The model under review builds one solid part; all positions refer to its coordinate system, in mm. A direction names the side the tool comes from. Round coordinates to 2 decimals unless told otherwise and drop trailing zeros. Order: outer loops, then holes, each group sorted by start corner. A loop starts at its lowest first (then second) coordinate and runs counter-clockwise, first axis right, second up. Notation, with made-up numbers: M 54.5,6.5 L 67.5,6.5 A24 cw 67.5,45.5 Z; hole C 69,24.25 d1. An arc over 180 degrees is marked long. One line per item, written item: value. Start each with the question number.
Autodesk Inventor part; units mm, degrees
ref_plane "YZ Plane" through (0, 0, 0) normal (1, 0, 0) x (0, 1, 0)
ref_plane "XZ Plane" through (0, 0, 0) normal (0, 1, 0) x (-1, 0, 0)
ref_plane "XY Plane" through (0, 0, 0) normal (0, 0, 1) x (1, 0, 0)
sketch "Sketch1" plane through (0, 0, 0) normal (0, 0, 1) x (1, 0, 0)
  line L0 (190, -75) -> (-250, -75)
  line L1 (190, 75) -> (190, -75)
  line L2 (-250, 75) -> (-235, 75)
  line L3 (-250, -75) -> (-250, 75)
  line L4 (-255, -10) -> (-255, -60)
  line L5 (-255, -60) -> (-250, -60)
  line L6 (-250, -10) -> (-250, -60)
  line L7 (-255, -10) -> (-250, -10)
  line L8 (-255, 60) -> (-255, 10)
  line L9 (-255, 10) -> (-250, 10)
  line L10 (-250, 60) -> (-250, 10)
  line L11 (-255, 60) -> (-250, 60)
  line L12 (190, 60) -> (190, 10)
  line L13 (190, 10) -> (195, 10)
  line L14 (195, 60) -> (195, 10)
  line L15 (190, 60) -> (195, 60)
  line L16 (190, -10) -> (190, -60)
  line L17 (190, -60) -> (195, -60)
  line L18 (195, -10) -> (195, -60)
  line L19 (190, -10) -> (195, -10)
  line L20 (140, 75) -> (152.5, 75)
  line L21 (20, -45) -> (55.3553, -9.6447)
  line L22 (-100, 75) -> (-78.9949, 53.9949)
  line L23 (-15.3553, -9.6447) -> (-18.8909, -13.1802)
  line L24 (-18.8909, -13.1802) -> (-40.1041, 8.033)
  line L25 (-40.1041, 8.033) -> (-36.5685, 11.5685)
  line L26 (-57.7817, 32.7817) -> (-36.5685, 11.5685)
  line L27 (-57.7817, 32.7817) -> (-61.3173, 29.2462)
  line L28 (-61.3173, 29.2462) -> (-82.5305, 50.4594)
  line L29 (-82.5305, 50.4594) -> (-78.9949, 53.9949)
  line L30 (118.9949, 53.9949) -> (140, 75)
  line L31 (118.9949, 53.9949) -> (122.5305, 50.4594)
  line L32 (122.5305, 50.4594) -> (101.3173, 29.2462)
  line L33 (101.3173, 29.2462) -> (97.7817, 32.7817)
  line L34 (76.5685, 11.5685) -> (97.7817, 32.7817)
  line L35 (76.5685, 11.5685) -> (80.1041, 8.033)
  line L36 (80.1041, 8.033) -> (58.8909, -13.1802)
  line L37 (58.8909, -13.1802) -> (55.3553, -9.6447)
  line L38 (-15.3553, -9.6447) -> (20, -45)
  line L39 (-210, 75) -> (-210, 70)
  line L40 (-210, 70) -> (-235, 70)
  line L41 (-235, 70) -> (-235, 75)
  line L42 (177.5, 75) -> (190, 75)
  line L43 (177.5, 75) -> (177.5, 70)
  line L44 (177.5, 70) -> (152.5, 70)
  line L45 (152.5, 70) -> (152.5, 75)
  line L46 (-165, 75) -> (-100, 75)
  line L47 (-165, 75) -> (-165, 70)
  line L48 (-165, 70) -> (-190, 70)
  line L49 (-190, 70) -> (-190, 75)
  line L50 (-210, 75) -> (-190, 75)
  point P0 (0, 0)
extrude "Extrusion1" add sketch "Sketch1" along normal blind 5
sketch "Sketch2" plane through (0, 0, 5) normal (0, 0, 1) x (1, 0, 0)
  point P0 (0, 0)
sketch "Sketch4" plane through (0, 0, 5) normal (0, 0, 1) x (1, 0, 0)
  line L0 (190, -60) -> (195, -60)
  line L1 (195, -60) -> (195, -10)
  line L2 (195, -10) -> (190, -10)
  line L3 (190, -10) -> (190, 10)
  line L4 (190, 10) -> (195, 10)
  line L5 (195, 10) -> (195, 60)
  line L6 (195, 60) -> (190, 60)
  line L7 (190, 60) -> (190, 75)
  line L8 (190, 75) -> (177.5, 75)
  line L9 (177.5, 75) -> (177.5, 70)
  line L10 (177.5, 70) -> (152.5, 70)
  line L11 (152.5, 70) -> (152.5, 75)
  line L12 (152.5, 75) -> (140, 75)
  line L13 (140, 75) -> (118.9949, 53.9949)
  line L14 (118.9949, 53.9949) -> (122.5305, 50.4594)
  line L15 (122.5305, 50.4594) -> (101.3173, 29.2462)
  line L16 (101.3173, 29.2462) -> (97.7817, 32.7817)
  line L17 (97.7817, 32.7817) -> (76.5685, 11.5685)
  line L18 (76.5685, 11.5685) -> (80.1041, 8.033)
  line L19 (80.1041, 8.033) -> (58.8909, -13.1802)
  line L20 (58.8909, -13.1802) -> (55.3553, -9.6447)
  line L21 (55.3553, -9.6447) -> (20, -45)
  line L22 (20, -45) -> (-15.3553, -9.6447)
  line L23 (-15.3553, -9.6447) -> (-18.8909, -13.1802)
  line L24 (-18.8909, -13.1802) -> (-40.1041, 8.033)
  line L25 (-40.1041, 8.033) -> (-36.5685, 11.5685)
  line L26 (-36.5685, 11.5685) -> (-57.7817, 32.7817)
  line L27 (-57.7817, 32.7817) -> (-61.3173, 29.2462)
  line L28 (-61.3173, 29.2462) -> (-82.5305, 50.4594)
  line L29 (-82.5305, 50.4594) -> (-78.9949, 53.9949)
  line L30 (-78.9949, 53.9949) -> (-100, 75)
  line L31 (-100, 75) -> (-165, 75)
  line L32 (-165, 75) -> (-165, 70)
  line L33 (-165, 70) -> (-190, 70)
  line L34 (-190, 70) -> (-190, 75)
  line L35 (-190, 75) -> (-210, 75)
  line L36 (-210, 75) -> (-210, 70)
  line L37 (-210, 70) -> (-235, 70)
  line L38 (-235, 70) -> (-235, 75)
  line L39 (-235, 75) -> (-250, 75)
  line L40 (-250, 75) -> (-250, 60)
  line L41 (-250, 60) -> (-255, 60)
  line L42 (-255, 60) -> (-255, 10)
  line L43 (-255, 10) -> (-250, 10)
  line L44 (-250, 10) -> (-250, -10)
  line L45 (-250, -10) -> (-255, -10)
  line L46 (-255, -10) -> (-255, -60)
  line L47 (-255, -60) -> (-250, -60)
  line L48 (-250, -60) -> (-250, -75)
  line L49 (-250, -75) -> (190, -75)
  line L50 (190, -75) -> (190, -60)
  line L51 (-140, -35) -> (-120, -35)
  line L52 (-120, -35) -> (-120, -55)
  line L53 (-120, -55) -> (-140, -55)
  line L54 (-140, -55) -> (-140, -35)
  point P0 (0, 0)
  dimension "d4" = 20
  dimension "d5" = 20
  dimension "d6" = 20
  dimension "d7" = 110
extrude "Extrusion3" cut sketch "Sketch4" against normal blind 10 contours L51 L52 L53 L54
properties part number "Fondo"
Item 1: Consider section C-C, the plane x = -4.5. Give the boundary of the cut face in (y, z), then the cut area to 4 significant figures.
Item 2: The part is to be moulded in two halves that separate along X. For faces 4 (the flat face through (-33, -16, 0)), 5 (the flat face through (-29.35, -2.72, 2.46)), 6 (the flat face through (-71.775, 39.704, 2.465)), say which applies: pulls with the +X half, pulls with the -X half, needs draft (parallel to the pull), parting line crosses it, or undercut.
Item 3: Machinability: for faces 1 (the flat face through (69.646, -2.425, 2.465)), 2 (the flat face through (-47, 22, 2)), 3 (the flat face through (-33, -16, 5)), which of the approach directions +Z, -Z, +X, -X, +Y, -Y give a long, thin tool a straight path to every point of the face, cutting with its end or side? Answer none if there is none.
Item 4: Consider section D-D, the plane x = 158. Give the boundary of the cut face in (y, z).
Item 5: Clearance check with flat-ended pins moving along their axes: P1, Ø1.5, axis at y = 73.5, z = 1.5, coming from the +X side; P2, Ø1.5, axis at x = -253.5, z = 2.5, coming from the -Y side; P3, Ø2.5, axis at x = -224.5, z = 2.5, coming from the +Y side. State where each tip first meets the part, or that it passes through.
Item 6: Wall thickness on L1, parallel to X at y = -53.5, z = 2.15; L2, parallel to X at y = -37, z = 2.45; L3, parallel to Y at x = 167, z = 4.6: over which ranges is each line inside the solid? List them lowest first.
Item 7: Consider section A-A, the plane y = -40.5. Give the boundary of the cut face in (x, z), then the cut area to 4 significant figures.
Item 8: Consider section B-B, the plane y = 1.5. Give the boundary of the cut face in (x, z).
Computed:
1. outline: M -75,0 L -20.5,0 L -20.5,5 L -75,5 Z
1. area: 272.5 mm^2
2. face 4: needs draft
2. face 5: undercut
2. face 6: undercut
3. face 1: +Z, -Z
3. face 2: +Z, -Z, +Y
3. face 3: +Z, +X, -X, +Y, -Y
4. outline: M -75,0 L 70,0 L 70,5 L -75,5 Z
5. P1: stops at x = 190
5. P2: stops at y = -60
5. P3: stops at y = 70
6. L1: x = -255 to -140, -120 to 195
6. L2: x = -255 to -140, -120 to 12, 28 to 195
6. L3: y = -75 to 70
7. outline: M -255,0 L -140,0 L -140,5 L -255,5 Z; M -120,0 L 15.5,0 L 15.5,5 L -120,5 Z; M 24.5,0 L 195,0 L 195,5 L 24.5,5 Z
7. area: 2,105 mm^2
8. outline: M -250,0 L -33.57,0 L -33.57,5 L -250,5 Z; M 73.57,0 L 190,0 L 190,5 L 73.57,5 Z
